from build123d import *

# Parameters (mm, degrees)
F1_DEPTH = 5
F0_R     = 1.3
F3_DEPTH = 5
F4_DEPTH = 5


with BuildPart() as f1:
    # F0 (on Top) → F1 (new body)
    with BuildSketch(Plane.XY):
        with BuildLine():
            ThreePointArc((25, 22.5), (23.232233047, 23.232233047), (22.5, 25))
            Line((22.5, 25), (-22.5, 25))
            ThreePointArc((-22.5, 25), (-23.232233047, 23.232233047), (-25, 22.5))
            Line((-25, 22.5), (-25, -22.5))
            ThreePointArc((-25, -22.5), (-23.232233047, -23.232233047), (-22.5, -25))
            Line((-22.5, -25), (22.5, -25))
            ThreePointArc((22.5, -25), (23.232233047, -23.232233047), (25, -22.5))
            Line((25, -22.5), (25, -2.5))
            Line((25, -2.5), (21, -2.5))
            Line((21, -2.5), (21, -21))
            Line((21, -21), (-21, -21))
            Line((-21, -21), (-21, 21))
            Line((-21, 21), (21, 21))
            Line((21, 21), (21, 2.5))
            Line((21, 2.5), (25, 2.5))
            Line((25, 2.5), (25, 22.5))
        make_face()
    extrude(amount=F1_DEPTH)



with BuildPart() as f1b:
    # F0 (on Top) → F1, piece 2 (new body)
    with BuildSketch(Plane.XY):
        with Locations((-17.5, 17.5)):
            Circle(F0_R)
    extrude(amount=F1_DEPTH)


with BuildPart() as f1c:
    # F0 (on Top) → F1, piece 3 (new body)
    with BuildSketch(Plane.XY):
        with Locations((-17.5, -17.5)):
            Circle(F0_R)
    extrude(amount=F1_DEPTH)


with BuildPart() as f1d:
    # F0 (on Top) → F1, piece 4 (new body)
    with BuildSketch(Plane.XY):
        with Locations((17.5, -17.5)):
            Circle(F0_R)
    extrude(amount=F1_DEPTH)


with BuildPart() as f1e:
    # F0 (on Top) → F1, piece 5 (new body)
    with BuildSketch(Plane.XY):
        with Locations((17.5, 17.5)):
            Circle(F0_R)
    extrude(amount=F1_DEPTH)


with BuildPart() as f1_1:
    add(f1.part)

    add(f1b.part)  # F3 merges F1b

    add(f1c.part)  # F3 merges F1c

    add(f1d.part)  # F3 merges F1d

    add(f1e.part)  # F3 merges F1e
    # F2 (on face) → F3 (join)
    with BuildSketch(Plane.XY):
        with BuildLine():
            Line((-22.5, -25), (22.5, -25))
            ThreePointArc((22.5, -25), (23.232233047, -23.232233047), (25, -22.5))
            Line((25, -22.5), (25, -2.5))
            Line((25, -2.5), (21, -2.5))
            Line((21, -2.5), (21, -21))
            Line((21, -21), (-21, -21))
            Line((-21, -21), (-21, 21))
            Line((-21, 21), (21, 21))
            Line((21, 21), (21, 2.5))
            Line((21, 2.5), (25, 2.5))
            Line((25, 2.5), (25, 22.5))
            ThreePointArc((25, 22.5), (23.232233047, 23.232233047), (22.5, 25))
            Line((22.5, 25), (-22.5, 25))
            ThreePointArc((-22.5, 25), (-23.232233047, 23.232233047), (-25, 22.5))
            Line((-25, 22.5), (-25, -22.5))
            ThreePointArc((-25, -22.5), (-23.232233047, -23.232233047), (-22.5, -25))
        make_face()
        Polygon((21, -2.5), (25, -2.5), (25, 2.5), (21, 2.5), (21, 21), (-21, 21), (-21, -21), (21, -21), align=None)
    extrude(amount=-F3_DEPTH)

    # F4 (add): a face of the model
    f4_faces = [f1_1.faces().sort_by_distance(p)[0] for p in [
        (22.732233047, 22.732233047, 5),
    ]]
    extrude(f4_faces, amount=F4_DEPTH)


solid = f1_1.part
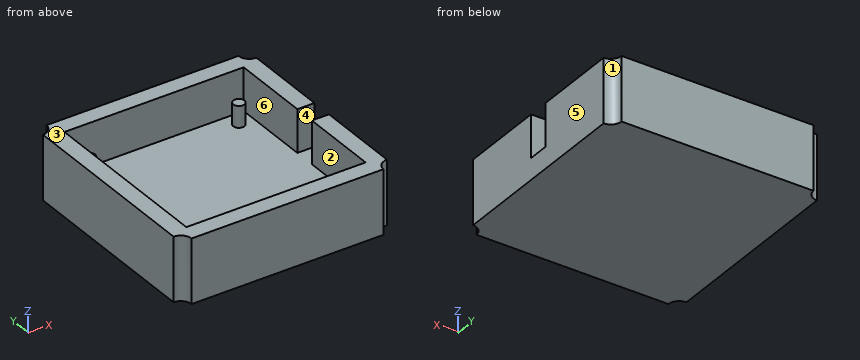
Build history of the part. All positions in model axes, mm. Face numbers are marked on the shaded views. A direction names the side the tool comes from. Give positions to 0.01 mm unless a question says otherwise; leave off trailing zeros. Loops run counter-clockwise (first coordinate to the right, second up) from the corner with the lowest first, then second, coordinate; pieces in that order, holes last. Notation, with made-up numbers: (39.5, -32.5) - (71.5, -32.5) arc R29 ccw to (71.5, -1.5) - close; hole circle Ø9 at (58.5, 43). An arc over 180 degrees is marked (long way). Write item = value, one per line. Start each with the question number.
1) Pull direction Y, two halves, no side cores. Call the marked faces 1, 2 and 3: +Y half, -Y half, draft (parallel to the pull), parting line (faces both ways), or undercut.
2) Probe probe 1 along Y at (x, z) = (-19, 5.75); probe 2 along Z at (x, y) = (-17.5, -17). List the from-to ranges inside material, lowest first. Write a range as from..to.
3) Band-saw the part on D-D on x = 8. Give the cut face in (y, z).
4) Band-saw the part on B-B on x = -17.5. Give the cut face in (y, z).
5) Band-saw the part on A-A on z = 3.5. Give the cut face in (x, y), plus the area to 3 significant figures.
6) Tool access for the marked faces 4, 5 and 6: list every direction of +Z, -Z, +X, -X, +Y, -Y with a clear straight run to the whole face (end or side of a thin tool).
7) Drop flat-ended pins along their axis: pin 1 Ø1.3 at (x, y) = (17.5, 17.5) entering from +Z; pin 2 Ø1.2 at (x, z) = (23.5, 3) entering from +Y. Give the stop position or say it passes through.
Final values:
q1.face_1 = +Y half
q1.face_2 = undercut
q1.face_3 = draft
q2.probe_1 = -25..-21, 21..25
q2.probe_2 = -5..5
q3.outline = (-25, -5) - (25, -5) - (25, 10) - (21, 10) - (21, 0) - (-21, 0) - (-21, 10) - (-25, 10) - close
q4.outline = (-25, -5) - (25, -5) - (25, 10) - (21, 10) - (21, 0) - (18.8, 0) - (18.8, 5) - (16.2, 5) - (16.2, 0) - (-16.2, 0) - (-16.2, 5) - (-18.8, 5) - (-18.8, 0) - (-21, 0) - (-21, 10) - (-25, 10) - close
q5.outline = (-25, -22.5) arc R2.5 cw to (-22.5, -25) - (22.5, -25) arc R2.5 cw to (25, -22.5) - (25, -2.5) - (21, -2.5) - (21, -21) - (-21, -21) - (-21, 21) - (21, 21) - (21, 2.5) - (25, 2.5) - (25, 22.5) arc R2.5 cw to (22.5, 25) - (-22.5, 25) arc R2.5 cw to (-25, 22.5) - close; circle Ø2.6 at (-17.5, -17.5); circle Ø2.6 at (-17.5, 17.5); circle Ø2.6 at (17.5, -17.5); circle Ø2.6 at (17.5, 17.5)
q5.area = 718 mm²
q6.face_4 = +Z, +X
q6.face_5 = +Z, -Z, +X, +Y, -Y
q6.face_6 = +Z
q7.pin_1 = 5
q7.pin_2 = 23.64
